Design review of the part built by this model. Coordinates are the model's own, in mm. Coordinates: 2 decimals unless noted, no trailing zeros. Loops run counter-clockwise (first coordinate to the right, second up) from the corner with the lowest first, then second, coordinate; pieces in that order, holes last. Notation, with made-up numbers: (-24.5, -12) - (-9.5, -12) arc R10 cw to (-9.5, -2) - close; hole circle Ø10 at (-27.75, 58). An arc over 180 degrees is marked (long way). Use one line per item in the form item = value. Start each with the question number.
(1) Add section A-A (y = -4.75). State the section outline as (x, z) points, plus the area to 3 significant figures.
(2) For L1, parallel to X at y = -2.1, z = 0; L2, parallel to X at y = -4, z = 1.5; L3, parallel to Z at x = 3.25, y = -2.75, list the stretches that pass through material, from the lowest coordinate up.
(3) Add section B-B (z = 0). State the section outline as (x, y) points, plus the area to 3 significant figures.
(4) The part is to be moulded in two halves that separate along Z. For faces 1 (the face through (0.1, 0, 6.2)), 2 (the face through (-4.01, -3.029, 3.075)), 3 (the face through (4.684, -2.958, 8.266)), say which applies: pulls with the +Z half, pulls with the -Z half, needs draft (parallel to the pull), parting line crosses it, or undercut.
(5) Clearance check with flat-ended pins moving along their axes: pin 1 Ø1 at (x, y) = (-4, -1.5) entering from +Z; pin 2 Ø1.5 at (x, y) = (-1, -4.5) entering from +Z; pin 3 Ø1.5 at (x, y) = (6.5, -3) entering from -Z. State where each tip first meets the part, or that it passes through.
```python
from build123d import *

# Parameters (mm, degrees)
SKETCH2_W               = 76
SKETCH2_H               = 76
CUT_EXTRUDE1_DEPTH      = 7
CUT_EXTRUDE1_DEPTH_BACK = 7


with BuildPart() as part:
    # Sketch1 → Revolve1 (revolve)
    with BuildSketch(Plane.XY):
        Polygon((0, 0), (9.45, 0), (20.646152423, -3), (9.45, -6), (0, -6), align=None)
    revolve(axis=Axis((0, -6, 0), (0, 1, 0)))

    # Sketch2 → Cut-Extrude1 (cut, two sides)
    with BuildSketch(Plane(origin=(0, 0, 0), x_dir=(1, 0, 0), z_dir=(0, 1, 0))) as cut_extrude1_sk:
        Rectangle(SKETCH2_W, SKETCH2_H)
        Polygon((-9.5, -5.484827557), (0, -10.969655115), (9.5, -5.484827557), (9.5, 5.484827557), (0, 10.969655115), (-9.5, 5.484827557), align=None, mode=Mode.SUBTRACT)
    extrude(amount=CUT_EXTRUDE1_DEPTH, mode=Mode.SUBTRACT)
    extrude(cut_extrude1_sk.sketch, amount=-CUT_EXTRUDE1_DEPTH_BACK, mode=Mode.SUBTRACT)

    # Sketch3 → Cut-Revolve1 (revolve, cut)
    with BuildSketch(Plane.XY):
        Polygon((0, 0), (6, 0), (5.053, -0.947), (5.053, -5.053), (6, -6), (0, -6), align=None)
    revolve(axis=Axis((0, -6, 0), (0, 1, 0)), mode=Mode.SUBTRACT)


solid = part.part
```
Computed values:
q1.outline = (-9.5, -5.48) - (0, -10.97) - (9.5, -5.48) - (9.5, 5.48) - (0, 10.97) - (-9.5, 5.48) - close; hole circle Ø10.11 at (0, 0)
q1.area = 232 mm^2
q2.L1 = -9.5 to -5.05, 5.05 to 9.5
q2.L2 = -9.5 to -4.83, 4.83 to 9.5
q2.L3 = -9.09 to -3.87, 3.87 to 9.09
q3.outline = (-9.5, -5.99) - (-9.45, -6) - (-6, -6) - (-5.05, -5.05) - (-5.05, -0.95) - (-6, 0) - (-9.45, 0) - (-9.5, -0.01) - close; (5.05, -5.05) - (6, -6) - (9.45, -6) - (9.5, -5.99) - (9.5, -0.01) - (9.45, 0) - (6, 0) - (5.05, -0.95) - close
q3.area = 51.6 mm^2
q4.face_1 = needs draft
q4.face_2 = undercut
q4.face_3 = pulls with the +Z half
q5.pin_1 = 8.95
q5.pin_2 = 10.83
q5.pin_3 = -7.65
